Design review of the part built by this model. Coordinates are the model's own, in mm. A direction names the side the tool comes from. Coordinates: 2 decimals unless noted, no trailing zeros. Write each loop counter-clockwise with the first axis right and the second up, starting at its lowest first coordinate (ties: lowest second). Pieces come first, ordered by that corner, then holes. Notation, with made-up numbers: M 49,-17.75 L 107,-17.75 A16 cw 107,-11.75 Z; hole C 14,64.25 d8. An arc over 180 degrees is marked long. Write item = value, one per line.
```python
from build123d import *

# Parameters (mm, degrees)
F0_W     = 106.1315912282
F0_H     = 74.4450837374
F0_W_2   = 98.5115912282
F0_H_2   = 66.8250837374
F1_DEPTH = 25.4
F0_R     = 9.0429354427
F2_DEPTH = 13.97
F3_DEPTH = 17.272
F4_D     = 3.5
F6_R     = 5.08


# Not quite as in the source:
# - a fillet or chamfer that OpenCascade refuses, or shapes differently, is made with other operations: its cross-section is extruded or revolved along the edge and cut away or added


with BuildPart() as f1:
    # F0 (on Top) → F1 (new body)
    with BuildSketch(Plane.XY):
        with Locations((0.6595404583, -2.4548470974)):
            Rectangle(F0_W, F0_H)
        with Locations((0.6595404583, -2.4548470974)):
            Rectangle(F0_W_2, F0_H_2, mode=Mode.SUBTRACT)
    extrude(amount=F1_DEPTH)

    # F0 (on Top) → F2 (join)
    with BuildSketch(Plane.XY):
        with Locations((0.6595404583, -2.4548470974)):
            Rectangle(F0_W_2, F0_H_2)
        with Locations((-26.1980332434, -15.4872145504)):
            Circle(F0_R, mode=Mode.SUBTRACT)
        with Locations((26.1980332434, -15.4872145504)):
            Circle(F0_R, mode=Mode.SUBTRACT)
        with Locations((-26.1980332434, 15.4872145504)):
            Circle(F0_R, mode=Mode.SUBTRACT)
        with Locations((26.1980332434, 15.4872145504)):
            Circle(F0_R, mode=Mode.SUBTRACT)
    extrude(amount=F2_DEPTH)

    # F0 (on Top) → F3 (join)
    with BuildSketch(Plane.XY):
        with Locations((-26.1980332434, -15.4872145504)):
            Circle(F0_R)
        with Locations((-26.1980332434, 15.4872145504)):
            Circle(F0_R)
        with Locations((26.1980332434, 15.4872145504)):
            Circle(F0_R)
        with Locations((26.1980332434, -15.4872145504)):
            Circle(F0_R)
    extrude(amount=F3_DEPTH)

    # F4 (through all)
    with Locations(Plane(origin=(0, 0, 0), x_dir=(1, 0, 0), z_dir=(0, 0, -1))):
        with Locations((0, 0)):
            Hole(F4_D / 2)

    # F5: chamfer of 5.08 on 4 edges, made by hand


with BuildPart() as f5_tool2:
    # F5_s3 → F5_t4 (revolve)
    with BuildSketch(Plane.XZ.offset(-15.4872145504)):
        Polygon((-17.1550978007, 12.192), (-22.2350978007, 17.272), (-17.1550978007, 17.272), align=None)
    revolve(axis=Axis((-26.1980332434, 15.4872145504, 17.272), (0, 0, 1)))

    split(bisect_by=Plane.XY.offset(13.97), keep=Keep.TOP)


with BuildPart() as f1_1:
    add(f1.part)

    # F5_t1: cut F5_tool2
    add(f5_tool2.part, mode=Mode.SUBTRACT)


with BuildPart() as f5_tool7:
    # F5_s8 → F5_t9 (revolve)
    with BuildSketch(Plane.XZ.offset(-15.4872145504)):
        Polygon((35.2409686861, 12.192), (30.1609686861, 17.272), (35.2409686861, 17.272), align=None)
    revolve(axis=Axis((26.1980332434, 15.4872145504, 17.272), (0, 0, 1)))

    split(bisect_by=Plane.XY.offset(13.97), keep=Keep.TOP)


with BuildPart() as f1_2:
    add(f1_1.part)

    # F5_t6: cut F5_tool7
    add(f5_tool7.part, mode=Mode.SUBTRACT)


with BuildPart() as f5_tool12:
    # F5_s13 → F5_t14 (revolve)
    with BuildSketch(Plane.XZ.offset(15.4872145504)):
        Polygon((35.2409686861, 12.192), (30.1609686861, 17.272), (35.2409686861, 17.272), align=None)
    revolve(axis=Axis((26.1980332434, -15.4872145504, 17.272), (0, 0, 1)))

    split(bisect_by=Plane.XY.offset(13.97), keep=Keep.TOP)


with BuildPart() as f1_3:
    add(f1_2.part)

    # F5_t11: cut F5_tool12
    add(f5_tool12.part, mode=Mode.SUBTRACT)


with BuildPart() as f5_tool17:
    # F5_s18 → F5_t19 (revolve)
    with BuildSketch(Plane.XZ.offset(15.4872145504)):
        Polygon((-17.1550978007, 12.192), (-22.2350978007, 17.272), (-17.1550978007, 17.272), align=None)
    revolve(axis=Axis((-26.1980332434, -15.4872145504, 17.272), (0, 0, 1)))

    split(bisect_by=Plane.XY.offset(13.97), keep=Keep.TOP)


with BuildPart() as f1_4:
    add(f1_3.part)

    # F5_t16: cut F5_tool17
    add(f5_tool17.part, mode=Mode.SUBTRACT)

    # F6
    f6_edges = [f1_4.edges().sort_by_distance(p)[0] for p in [
        (-52.406255, -39.677389, 12.7),
        (-52.406255, 34.767695, 12.7),
        (53.725336, -39.677389, 12.7),
        (53.725336, 34.767695, 12.7),
    ]]
    fillet(f6_edges, radius=F6_R)


solid = f1_4.part
```
Q1. The part is to be moulded in two halves that separate along Y. For faces 3 (the flat face through (-52.406, -3, 13)), 4 (the cylindrical face through (-50.96, -38.15, 12.88)), 5 (the flat face through (-48.596, -3, 20)), 6 (the flat face through (0, -2, 13.97)), say which applies: +Y half, -Y half, draft (parallel to the pull), parting line (faces both ways), or undercut.
Check result:
face_3 = draft
face_4 = -Y half
face_5 = undercut
face_6 = undercut
Q2. Wall thickness on line 1 (X direction, y = 14, z = 15.5); line 2 (Y direction, x = 48.5, z = 21); line 3 (Y direction, x = 0, z = 6): over which ranges is each line inside the solid? List them lowest first.
Check result:
line_1 = -52.41 to -48.6, -31.74 to -20.66, 20.66 to 31.74, 49.92 to 53.73
line_2 = -39.68 to -35.87, 30.96 to 34.77
line_3 = -39.68 to -1.75, 1.75 to 34.77
Q3. Consider section D-D, the plane z = 16. State the section outline as (x, y) points.
Check result:
outline = M -52.41,-34.6 A5.08 ccw -47.33,-39.68 L 48.65,-39.68 A5.08 ccw 53.73,-34.6 L 53.73,29.69 A5.08 ccw 48.65,34.77 L -47.33,34.77 A5.08 ccw -52.41,29.69 Z; C -26.2,-15.49 d10.47; C -26.2,15.49 d10.47; C 26.2,-15.49 d10.47; C 26.2,15.49 d10.47; hole M -48.6,-35.87 L 49.92,-35.87 L 49.92,30.96 L -48.6,30.96 Z
Q4. Consider section C-C, the plane y = 0. State the section outline as (x, z) points, and give its area (3 significant figures).
Check result:
outline = M -52.41,0 L -1.75,0 L -1.75,13.97 L -48.6,13.97 L -48.6,25.4 L -52.41,25.4 Z; M 1.75,0 L 53.73,0 L 53.73,25.4 L 49.92,25.4 L 49.92,13.97 L 1.75,13.97 Z
area = 1,520 mm²
Q5. For P1, Ø2.5, axis at x = 27, y = 16, coming from the +Z side; P2, Ø5, axis at x = 20, y = -13, coming from the +Z side; P3, Ø6, axis at x = 32, y = 20.5, coming from the +Z side, all flat-tipped, find the tip position at first contact; note any pin that passes through.
Check result:
P1 = 17.27
P2 = 17.06
P3 = 16.57
Q6. Consider section B-B, the plane z = 22. State the section outline as (x, y) points, and give its area (3 significant figures).
Check result:
outline = M -52.41,-34.6 A5.08 ccw -47.33,-39.68 L 48.65,-39.68 A5.08 ccw 53.73,-34.6 L 53.73,29.69 A5.08 ccw 48.65,34.77 L -47.33,34.77 A5.08 ccw -52.41,29.69 Z; hole M -48.6,-35.87 L 49.92,-35.87 L 49.92,30.96 L -48.6,30.96 Z
area = 1,300 mm²
Q7. Machinability: for faces 1 (the cylindrical face through (-1.617, 0.67, 7.083)), 2 (the flat face through (49.915, -3, 20)), which of the approach directions +Z, -Z, +X, -X, +Y, -Y give a long, thin tool a straight path to every point of the face, cutting with its end or side? Answer none if there is none.
Check result:
face_1 = +Z, -Z
face_2 = +Z
Q8. Consider section A-A, the plane x = 0. State the section outline as (y, z) points, and give its area (3 significant figures).
Check result:
outline = M -39.68,0 L -1.75,0 L -1.75,13.97 L -35.87,13.97 L -35.87,25.4 L -39.68,25.4 Z; M 1.75,0 L 34.77,0 L 34.77,25.4 L 30.96,25.4 L 30.96,13.97 L 1.75,13.97 Z
area = 1,080 mm²
